Check sheet for the modelled part. Datum: model origin and axes. Units: mm. Give positions to 0.01 mm unless a question says otherwise; leave off trailing zeros. Write each loop counter-clockwise with the first axis right and the second up, starting at its lowest first coordinate (ties: lowest second). Pieces come first, ordered by that corner, then holes. Notation, with made-up numbers: (-27, 24.25) -> (32, 24.25) arc R26 ccw to (32, 45.25) -> close; hole circle Ø3 at (-22, 77). An arc over 180 degrees is marked (long way). Use a Markdown table: item, result. Add a question column.
1. Cross-section at A-A (x = -5). Enter the section's corners in (y, z), then the cut area to 3 significant figures.
2. Scan lines: probe 1 along Y at (x, z) = (-14.5, 4.5); probe 2 along Z at (x, y) = (-11, 35.5); probe 3 along Y at (x, z) = (-9, -7.5). Record each from-to range of solid material in increasing order. Write a range as [from, to].
3. Gauge pin test, flat end, axial feed: P1, Ø1, axis at x = -8, z = 4, coming from the +Y side. Record the tip position at first contact, or that the pin passes through.
4. Cross-section at C-C (y = 34.5). Enter the section's corners in (x, z), then the cut area to 3 significant figures.
5. Cross-section at B-B (z = -9.5). Enter the section's corners in (x, y), then the cut area to 3 significant figures.
from build123d import *

# Parameters (mm, degrees)
SALIENTE_EXTRUIR4_DEPTH = 16.5


with BuildPart() as part:
    # Croquis1 → Saliente-Extruir4 (new, symmetric)
    with BuildSketch(Plane(origin=(0, 0, 0), x_dir=(0, 0, -1), z_dir=(1, 0, 0))):
        with BuildLine():
            Line((-12, -30), (12, -30))
            ThreePointArc((12, -30), (12.707106781, -29.707106781), (13, -29))
            Line((13, -29), (13, 29))
            ThreePointArc((13, 29), (0, 42), (-13, 29))
            Line((-13, 29), (-13, -29))
            ThreePointArc((-13, -29), (-12.707106781, -29.707106781), (-12, -30))
        make_face()
    extrude(amount=SALIENTE_EXTRUIR4_DEPTH, both=True)


solid = part.part
Worked answers:
| question | item | result |
|---|---|---|
| 1 | outline | (-30, -12) arc R1 ccw to (-29, -13) -> (29, -13) arc R13 ccw to (29, 13) -> (-29, 13) arc R1 ccw to (-30, 12) -> close |
| 1 | area | 1,800 mm² |
| 2 | probe 1 | y = [-30, 41.2] |
| 2 | probe 2 | z = [-11.26, 11.26] |
| 2 | probe 3 | y = [-30, 39.62] |
| 3 | P1 | stops at y = 41.52 |
| 4 | outline | (-16.5, -11.78) -> (16.5, -11.78) -> (16.5, 11.78) -> (-16.5, 11.78) -> close |
| 4 | area | 777 mm² |
| 5 | outline | (-16.5, -30) -> (16.5, -30) -> (16.5, 37.87) -> (-16.5, 37.87) -> close |
| 5 | area | 2,240 mm² |
